Could you check a few things on this model? Use its own coordinates, in mm. Face numbers are marked on the shaded views. A direction names the side the tool comes from. Give positions to 0.01 mm unless a question says otherwise; leave off trailing zeros. Order: outer loops, then holes, each group sorted by start corner. A loop starts at its lowest first (then second) coordinate and runs counter-clockwise, first axis right, second up. Notation, with made-up numbers: M 80.25,71 L 131.25,71 A22 ccw 131.25,77 Z; hole C -35.75,32 d8. An arc over 180 degrees is marked long. Answer in a Markdown table with one row per item. Add a question column.
Autodesk Inventor part; units mm, degrees
ref_plane "YZ Plane" through (0, 0, 0) normal (1, 0, 0) x (0, 1, 0)
ref_plane "XZ Plane" through (0, 0, 0) normal (0, 1, 0) x (-1, 0, 0)
ref_plane "XY Plane" through (0, 0, 0) normal (0, 0, 1) x (1, 0, 0)
ref_plane "Work Plane1" through (0, 0, 0) normal (0, 0, 1) x (1, 0, 0)
sketch "Sketch1" plane through (0, 0, 0) normal (0, 0, 1) x (1, 0, 0)
  line L0 (-41.9, 57.6) -> (-41.9, 91.9) construction
  line L1 (-41.9, -91.9) -> (41.9, -91.9) construction
  line L2 (-7.4, -59.4) -> (-7.4, -67.3) construction
  circle A0 centre (-24.65, -74.65) radius 17.25 construction
  circle A1 centre (-24.65, -74.65) radius 6.3062 construction
  circle A2 centre (-24.65, -74.65) radius 1.9
  line L3 (-24.65, -74.65) -> (11.6672, -38.3328) construction
  line L4 (-17.5789, -81.7211) -> (18.7383, -45.4039)
  line L5 (4.5961, -31.2617) -> (-31.7211, -67.5789)
  arc A3 (-31.7211, -67.5789) -> (-17.5789, -81.7211) centre (-24.65, -74.65) ccw
  arc A4 (18.7383, -45.4039) -> (4.5961, -31.2617) centre (11.6672, -38.3328) ccw construction
  circle A5 centre (11.6672, -38.3328) radius 2.6562
  line L6 (4.5961, -31.2617) -> (12.137, -23.7208)
  line L7 (3.5996, -14.8432) -> (9.3348, -8.7305) construction
  line L8 (33.237, -42.6502) -> (38.9722, -36.5375) construction
  line L9 (12.137, -23.7208) -> (33.5765, -45.1603) construction
  line L10 (33.5765, -45.1603) -> (12.137, -23.7208)
  line L11 (18.7383, -45.4039) -> (29.8258, -56.4914)
  line L12 (29.8258, -56.4914) -> (44.5482, -41.7691)
  line L13 (44.5482, -41.7691) -> (40.758, -37.9789)
  line L14 (40.758, -37.9789) -> (33.5765, -45.1603)
  point P0 (0, 0)
  point P1 (41.9, -91.9)
  point P2 (-6.4914, -56.4914)
  dimension "d0" = 3.8
  dimension "d3" = 10
  dimension "d4" = 45
  dimension "d5" = 40.64
  dimension "d6" = 20.32
extrude "Extrusion1" add sketch "Sketch1" along normal blind 10
sketch "Sketch2" plane through (0, 0, 10) normal (0, 0, 1) x (1, 0, 0)
  circle A0 centre (-24.65, -74.65) radius 1.9
  circle A1 centre (11.6672, -38.3328) radius 2.6562
  line L0 (-17.5789, -81.7211) -> (18.7383, -45.4039)
  line L1 (18.7383, -45.4039) -> (29.8258, -56.4914)
  line L2 (29.8258, -56.4914) -> (44.5482, -41.7691)
  line L3 (44.5482, -41.7691) -> (40.758, -37.9789)
  line L4 (40.758, -37.9789) -> (33.5765, -45.1603)
  line L5 (33.5765, -45.1603) -> (12.137, -23.7208)
  line L6 (12.137, -23.7208) -> (-31.7211, -67.5789)
  arc A2 (-31.7211, -67.5789) -> (-17.5789, -81.7211) centre (-24.65, -74.65) ccw
  line L7 (44.5482, -41.7691) -> (40.758, -37.9789)
  line L8 (44.5482, -41.7691) -> (40.758, -37.9789)
  line L9 (40.758, -37.9789) -> (26.0356, -52.7012)
  line L10 (26.0356, -52.7012) -> (29.8258, -56.4914)
  line L11 (29.8258, -56.4914) -> (44.5482, -41.7691)
  line L12 (18.7383, -45.4039) -> (29.8258, -56.4914)
  line L13 (26.0356, -52.7012) -> (18.7383, -45.4039)
  line L14 (18.7383, -45.4039) -> (26.2792, -37.863)
  line L15 (26.2792, -37.863) -> (33.5765, -45.1603)
  line L16 (33.5765, -45.1603) -> (26.0356, -52.7012)
  point P0 (0, 0)
extrude "Extrusion2" add sketch "Sketch2" along normal blind 25.4 contours L14 L5 L9 L1 | L9 L4 L3 L2 L1
sketch "Sketch3" plane through (44.5482, -41.7691, 35.4) normal (0.7071068, -0.7071068, 0) x (-0.7071068, -0.7071068, 0)
  circle A0 centre (5.6027, 15.08) radius 1.25
  line L0 (20.8205, 35.4) -> (0, 35.4)
  point P0 (1.9651, 35.4)
  dimension "d9" = 2.5
  dimension "d10" = 20.32
extrude "Extrusion3" cut sketch "Sketch3" against normal blind 25.4
sketch "Sketch4" plane through (-17.5789, -81.7211, 10) normal (0.7071068, -0.7071068, 0) x (-0.7071068, -0.7071068, 0)
  line L0 (10, 10) -> (10, 0)
  line L1 (10, 7.3414) -> (-12.1363, 7.3414)
  line L2 (-14.7676, 5.9432) -> (-18.7808, 0)
  line L3 (0, 0) -> (-51.3603, 0)
  arc A0 (-12.1363, 7.3414) -> (-14.7676, 5.9432) centre (-12.1363, 4.1664) ccw
  line L4 (-18.7808, 0) -> (10, 0)
  line L5 (10, 7.3414) -> (10, 0)
  point P0 (-70.2157, 10)
  dimension "d13" = 3.175
extrude "Extrusion4" cut sketch "Sketch4" against normal blind 25.4
properties part number "30_CUBE_openSIM_Laserarm"
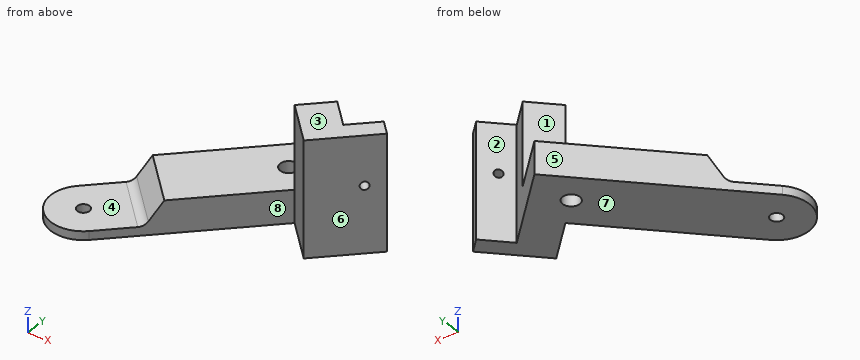
1. Suppose I cut it at B-B on z = 15. List the corners of the cut face in (x, y) for me.
2. Suppose I cut it at C-C on y = -74.65. List the corners of the cut face in (x, z) for me.
3. Suppose I cut it at A-A on x = -25. List the corners of the cut face in (y, z) for me, plus the area to 3 significant figures.
4. Will these pins go through, and if not, where does the flat tip stop? P1, Ø2.5, axis at x = -24.65, y = -74.65, coming from the +Z side; P2, Ø6, axis at x = 11.67, y = -38.33, coming from the +Z side; P3, Ø10, axis at y = -48, z = 12, coming from the -X side; P4, Ø4, axis at x = 29, z = 26.5, coming from the +Y side.
5. For the marked faces 1, 2, 3, 4 and 5, which set-ups out of +Z, -Z, +X, -X, +Y, -Y let a thin tool reach every point of the face, with its end or its side?
6. Thinking about a two-plate mould opening in X: for the marked faces 6, 7 and 8, which applies, pulls with the +X half, pulls with the -X half, needs draft (parallel to the pull), parting line crosses it, or undercut?
7. If I drill on line 1 along X through (y, z) = (-74, 2); line 2 along Y through (x, z) = (-24.65, 0.8); line 3 along X through (y, z) = (-40, 11.5), over which ranges is the centre line in solid material (lowest first)? Write a range as [from, to].
8. Suppose I cut it at D-D on x = 23.5. List the corners of the cut face in (y, z) for me.
Findings below:
| question | item | result |
|---|---|---|
| 1 | outline | M 18.74,-45.4 L 29.83,-56.49 L 44.55,-41.77 L 40.76,-37.98 L 33.58,-45.16 L 26.28,-37.86 Z |
| 2 | outline | M -34.65,0 L -26.55,0 L -26.55,2.66 L -34.65,2.66 Z; M -22.75,0 L -10.51,0 L -10.51,2.66 L -22.75,2.66 Z |
| 3 | outline | M -84.64,0 L -76.52,0 L -76.52,2.66 L -84.64,2.66 Z; M -72.78,0 L -60.86,0 L -60.86,2.66 L -72.78,2.66 Z |
| 3 | area | 53.3 mm2 |
| 4 | P1 | through |
| 4 | P2 | z = 10 |
| 4 | P3 | x = -16.72 |
| 4 | P4 | y = -38.58 |
| 5 | face 1 | +Z, -X, +Y |
| 5 | face 2 | +Z, -Z, +Y |
| 5 | face 3 | +Z, +X, -X, +Y, -Y |
| 5 | face 4 | +Z, -X, -Y |
| 5 | face 5 | +Z, -Z, -X, +Y |
| 6 | face 6 | pulls with the +X half |
| 6 | face 7 | needs draft |
| 6 | face 8 | undercut |
| 7 | line 1 | [-34.63, -26.44], [-22.86, -9.86] |
| 7 | line 2 | [-84.65, -76.55], [-72.75, -60.51] |
| 7 | line 3 | [24.14, 28.42], [38.74, 42.78] |
| 8 | outline | M -50.17,0 L -35.08,0 L -35.08,10 L -40.64,10 L -40.64,35.4 L -50.17,35.4 Z |
